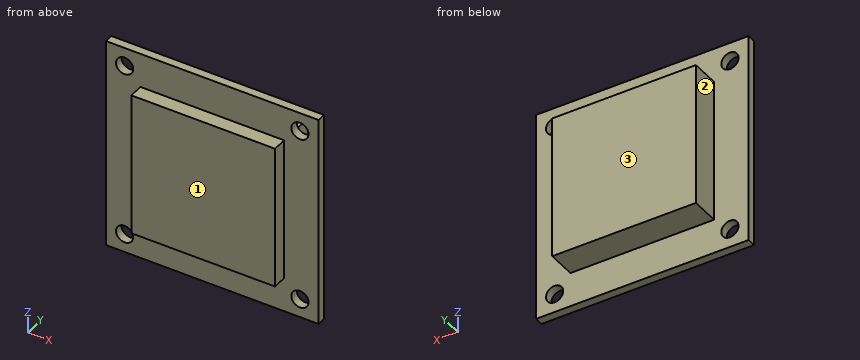
```python
from build123d import *

# Parameters (mm, degrees)
SKETCH_1_W           = 37
SKETCH_1_H           = 37
SKETCH_1_R           = 1.5
EXTRUDE_1_DEPTH      = 1.5
EXTRUDE_2_DEPTH      = 5
EXTRUDE_2_DEPTH_BACK = 4
SKETCH_2_W           = 25
SKETCH_2_H           = 25


with BuildPart() as part:
    # 草图1 → 凸台-拉伸1 (new body)
    with BuildSketch(Plane(origin=(0, 0, 0), x_dir=(1, 0, 0), z_dir=(0, 1, 0))):
        Rectangle(SKETCH_1_W, SKETCH_1_H)
        with Locations(Location((-15.25, 15.25, 0), (0, 0, 270))):
            Circle(SKETCH_1_R, mode=Mode.SUBTRACT)
        with Locations(Location((15.25, 15.25, 0), (0, 0, 270))):
            Circle(SKETCH_1_R, mode=Mode.SUBTRACT)
        with Locations(Location((15.25, -15.25, 0), (0, 0, 270))):
            Circle(SKETCH_1_R, mode=Mode.SUBTRACT)
        with Locations(Location((-15.25, -15.25, 0), (0, 0, 270))):
            Circle(SKETCH_1_R, mode=Mode.SUBTRACT)
    extrude(amount=EXTRUDE_1_DEPTH)

    # 草图2 → 凸台-拉伸2 (add, two sides: drawn at the far end of the back side and taken through both)
    with BuildSketch(Plane(origin=(0, 1.5, 0), x_dir=(1, 0, 0), z_dir=(0, 1, 0)).offset(-EXTRUDE_2_DEPTH_BACK)):
        Rectangle(SKETCH_2_W, SKETCH_2_H)
    extrude(amount=EXTRUDE_2_DEPTH + EXTRUDE_2_DEPTH_BACK)


solid = part.part
```
Input: part model. Units: mm. Frame: model coordinates. Face numbers are marked on the shaded views. Give positions to 0.01 mm unless a question says otherwise; leave off trailing zeros. Loops run counter-clockwise (first coordinate to the right, second up) from the corner with the lowest first, then second, coordinate; pieces in that order, holes last. Notation, with made-up numbers: (9, -29.75) -> (27, -29.75) arc R16 cw to (27, -6.75) -> close; hole circle Ø5 at (42.25, 30). An arc over 180 degrees is marked (long way). Use a Markdown table: item, result.
Q1. Section query A-A, the plane x = -15.25. Return the cut outline in (y, z), plus the area to 3 significant figures.
Entries:
| item | result |
|---|---|
| outline | (0, -18.5) -> (1.5, -18.5) -> (1.5, -16.75) -> (0, -16.75) -> close; (0, -13.75) -> (1.5, -13.75) -> (1.5, 13.75) -> (0, 13.75) -> close; (0, 16.75) -> (1.5, 16.75) -> (1.5, 18.5) -> (0, 18.5) -> close |
| area | 46.5 mm² |
Q2. Pull-direction query (Y, two-part tool) for the marked faces 1, 2 and 3; classes: pulls with the +Y half, pulls with the -Y half, needs draft (parallel to the pull), parting line crosses it, or undercut.
Entries:
| item | result |
|---|---|
| face 1 | pulls with the -Y half |
| face 2 | needs draft |
| face 3 | pulls with the +Y half |
Q3. Section query D-D, the plane z = -3.5. Return the cut outline in (x, y), plus the area to 3 significant figures.
Entries:
| item | result |
|---|---|
| outline | (-18.5, 0) -> (-12.5, 0) -> (-12.5, -2.5) -> (12.5, -2.5) -> (12.5, 0) -> (18.5, 0) -> (18.5, 1.5) -> (12.5, 1.5) -> (12.5, 6.5) -> (-12.5, 6.5) -> (-12.5, 1.5) -> (-18.5, 1.5) -> close |
| area | 243 mm² |
Q4. Ray query, probe 1 along X at (y, z) = (1, -15.25); probe 2 along X at (y, z) = (1, -16); probe 3 along Y at (x, z) = (16.5, -14). Return the intervals inside material, ascending. Write a range as from..to.
Entries:
| item | result |
|---|---|
| probe 1 | x = -18.5..-16.75, -13.75..13.75, 16.75..18.5 |
| probe 2 | x = -18.5..-16.55, -13.95..13.95, 16.55..18.5 |
| probe 3 | y = 0..1.5 |
Q5. Section query B-B, the plane z = -15.25. Return the cut outline in (x, y).
Entries:
| item | result |
|---|---|
| outline | (-18.5, 0) -> (-16.75, 0) -> (-16.75, 1.5) -> (-18.5, 1.5) -> close; (-13.75, 0) -> (13.75, 0) -> (13.75, 1.5) -> (-13.75, 1.5) -> close; (16.75, 0) -> (18.5, 0) -> (18.5, 1.5) -> (16.75, 1.5) -> close |
Q6. First-contact query: P1, Ø5, axis at x = 15.25, z = 15.25, coming from the +Y side; P2, Ø1.8, axis at x = -15.25, z = 15.25, coming from the -Y side; P3, Ø2, axis at x = 6, y = -1.5, coming from the +Z side; P4, Ø4, axis at x = -1, y = 5, coming from the -Z side. Flat tips, straight axial feed; report the tip coordinate or a pass-through.
Entries:
| item | result |
|---|---|
| P1 | stops at y = 1.5 |
| P2 | passes through |
| P3 | stops at z = 12.5 |
| P4 | stops at z = -12.5 |
Q7. Section query C-C, the plane y = 1. Return the cut outline in (x, z), plus the area to 3 significant figures.
Entries:
| item | result |
|---|---|
| outline | (-18.5, -18.5) -> (18.5, -18.5) -> (18.5, 18.5) -> (-18.5, 18.5) -> close; hole circle Ø3 at (-15.25, -15.25); hole circle Ø3 at (-15.25, 15.25); hole circle Ø3 at (15.25, -15.25); hole circle Ø3 at (15.25, 15.25) |
| area | 1,340 mm² |
